Geometry: final body of the model. Coordinates: model frame, mm. Face numbers are marked on the shaded views. A direction names the side the tool comes from. Coordinates: 2 decimals unless noted, no trailing zeros. Write each loop counter-clockwise with the first axis right and the second up, starting at its lowest first coordinate (ties: lowest second). Pieces come first, ordered by that corner, then holes. Notation, with made-up numbers: (7, 60) - (22, 60) arc R27 cw to (22, 89) - close; hole circle Ø4 at (61, -2). An arc over 180 degrees is marked (long way). Put each result on its own line as item: value.
```python
from build123d import *

# Parameters (mm, degrees)
F0_W     = 127
F0_H     = 78.5267129702
F1_DEPTH = 32.512
F2_T     = -2.54


# Not quite as in the source:
# - a feature of the source that left no trace in its solid (it failed there, or was rolled back) is left out


with BuildPart() as f1:
    # F0 (on Front) → F1 (new body)
    with BuildSketch(Plane.XZ):
        with Locations((-42.0160433277, -23.7329155207)):
            Rectangle(F0_W, F0_H)
    extrude(amount=F1_DEPTH)

    # F2
    f2_openings = [f1.faces().sort_by_distance(p)[0] for p in [
        (21.483957, -16.256, -23.732916),
        (-42.016043, -16.256, -62.996272),
        (-42.016043, 0, -23.732916),
    ]]
    offset(amount=F2_T, openings=f2_openings)


solid = f1.part
```
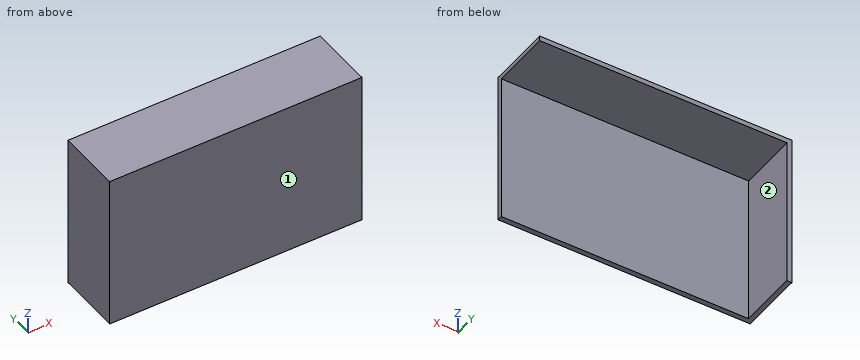
1. Section query B-B (y = -18.5). Return loops of the section in (x, z).
Answer below:
outline: (-105.52, -63) - (-102.98, -63) - (-102.98, 12.99) - (21.48, 12.99) - (21.48, 15.53) - (-105.52, 15.53) - close
2. Section query A-A (x = 13). Return loops of the section in (y, z), then the cut area to 3 significant figures.
Answer below:
outline: (-32.51, -63) - (-29.97, -63) - (-29.97, 12.99) - (0, 12.99) - (0, 15.53) - (-32.51, 15.53) - close
area: 276 mm²
3. Ray query, probe 1 along X at (y, z) = (-26.5, -48); probe 2 along Y at (x, z) = (-56, -14.5); probe 3 along Z at (x, y) = (-80, -0.5). Return the intervals inside material, ascending. Write a range as from..to.
Answer below:
probe 1: x = -105.52..-102.98
probe 2: y = -32.51..-29.97
probe 3: z = 12.99..15.53
4. Set-up query: the marked faces 1 and 2. Return all of +Z, -Z, +X, -X, +Y, -Y with unobstructed straight access to the full face (end or side cutting, diameter ignored); none if empty.
Answer below:
face 1: +Z, -Z, +X, -X, -Y
face 2: -Z, +X, +Y
5. Pin query (flat end, axial travel): pin 1 Ø1 at (x, z) = (1.5, -51) entering from +Y; pin 2 Ø4 at (x, y) = (-67, -16) entering from -Z; pin 3 Ø15 at (y, z) = (-10.5, -19) entering from +X. Return the tip coordinate at first contact, or that it passes through.
Answer below:
pin 1: stops at y = -29.97
pin 2: stops at z = 12.99
pin 3: stops at x = -102.98
